```python
from build123d import *

# Parameters (mm, degrees)
BOSS_EXTRUDE1_DEPTH = 1.5875
CUT_EXTRUDE2_DEPTH  = 93.054574745
FILLET1_R           = 2.54
FILLET2_R           = 1.27
FILLET3_R           = 0.508
FILLET4_R           = 0.508
BOSS_EXTRUDE3_DEPTH = 1.5875
FILLET5_R           = 1.27
FILLET6_R           = 0.254
BOSS_EXTRUDE4_DEPTH = 1.5875
CUT_EXTRUDE1_REACH  = 94.055
FILLET9_R           = 1.27
FILLET10_R          = 0.381
FILLET12_R          = 1.27
FILLET13_R          = 0.508


with BuildPart() as part:
    # Sketch1 → Boss-Extrude1 (new body)
    with BuildSketch(Plane(origin=(0, 0, 0), x_dir=(0, 0, -1), z_dir=(1, 0, 0))):
        with BuildLine():
            Line((62.185099246, -6.2738), (85.344, -14.722370106))
            Line((85.344, -14.722370106), (88.3158, -14.722370106))
            ThreePointArc((88.3158, -14.722370106), (90.111851224, -13.978421331), (90.8558, -12.182370106))
            Line((90.8558, -12.182370106), (90.8558, -12.131570106))
            Line((90.8558, -12.131570106), (89.3826, -10.658370106))
            Line((89.3826, -10.658370106), (88.9508, -10.658370106))
            Line((88.9508, -10.658370106), (88.9508, -12.182370106))
            Line((88.9508, -12.182370106), (87.376, -12.182370106))
            Line((87.376, -12.182370106), (87.376, -10.277370106))
            Line((87.376, -10.277370106), (85.344, -10.277370106))
            Line((85.344, -10.277370106), (85.344, -11.477881212))
            Line((85.344, -11.477881212), (71.07876946, -6.2738))
            Line((71.07876946, -6.2738), (87.376, -6.2738))
            Line((87.376, -6.2738), (87.376, 6.867629894))
            Line((87.376, 6.867629894), (88.9508, 6.867629894))
            Line((88.9508, 6.867629894), (88.9508, 5.089629894))
            Line((88.9508, 5.089629894), (89.9668, 5.089629894))
            ThreePointArc((89.9668, 5.089629894), (90.595417928, 5.350011965), (90.8558, 5.978629894))
            Line((90.8558, 5.978629894), (90.8558, 6.359629894))
            ThreePointArc((90.8558, 6.359629894), (90.111851224, 8.155681118), (88.3158, 8.899629894))
            Line((88.3158, 8.899629894), (85.344, 8.899629894))
            Line((85.344, 8.899629894), (62.185099246, 2.453000952))
            Line((62.185099246, 2.453000952), (-5.3213, 6.613676867))
            Line((-5.3213, 6.613676867), (-5.3213, 8.924406911))
            Line((-5.3213, 8.924406911), (-7.8613, 8.924406911))
            Line((-7.8613, 8.924406911), (-7.8613, 4.225406911))
            Line((-7.8613, 4.225406911), (-3.7338, 3.971013401))
            Line((-3.7338, 3.971013401), (-3.7338, 3.488413401))
            Line((-3.7338, 3.488413401), (-1.331252938, 3.488413401))
            ThreePointArc((-1.331252938, 3.488413401), (3.7338, 0), (-1.331252938, -3.488413401))
            Line((-1.331252938, -3.488413401), (-3.7338, -3.488413401))
            Line((-3.7338, -3.488413401), (-3.7338, -3.7338))
            Line((-3.7338, -3.7338), (-5.3213, -3.7338))
            Line((-5.3213, -3.7338), (-7.8613, -3.7338))
            Line((-7.8613, -3.7338), (-7.8613, -8.4328))
            Line((-7.8613, -8.4328), (-5.3213, -8.4328))
            Line((-5.3213, -8.4328), (-5.3213, -6.2738))
            Line((-5.3213, -6.2738), (62.185099246, -6.2738))
        make_face()
        Polygon((12.4587, -3.7338), (6.2738, -3.7338), (6.2738, 3.354206983), (12.4587, 2.973008093), align=None, mode=Mode.SUBTRACT)
        Polygon((14.3637, -4.3688), (14.3637, 3.495415512), (37.420099246, 2.074362011), (37.420099246, -4.3688), align=None, mode=Mode.SUBTRACT)
        Polygon((64.471099246, -4.3688), (64.471099246, 0.407106085), (85.344, -0.879370106), (85.344, -4.3688), align=None, mode=Mode.SUBTRACT)
        Polygon((39.325099246, -4.3688), (39.325099246, 1.956949622), (62.185099246, 0.548000952), (62.185099246, -4.3688), align=None, mode=Mode.SUBTRACT)
        Polygon((85.344, 6.922200335), (85.344, 1.025629894), (68.00108793, 2.094539469), align=None, mode=Mode.SUBTRACT)
    extrude(amount=BOSS_EXTRUDE1_DEPTH)

    # Sketch7 → Cut-Extrude2 (cut, through all)
    with BuildSketch(Plane.ZY):
        Polygon((6.5913, 8.924406911), (7.8613, 5.495406911), (7.8613, 8.924406911), align=None)
        Polygon((6.5913, -8.4328), (7.8613, -5.0038), (7.8613, -8.4328), align=None)
    extrude(amount=-CUT_EXTRUDE2_DEPTH, mode=Mode.SUBTRACT)

    # Fillet1
    fillet1_edges = [part.edges().sort_by_distance(p)[0] for p in [
        (0.79375, 2.453000952, -62.185099246),
        (0.79375, 8.899629894, -85.344),
        (0.79375, -14.722370106, -85.344),
        (0.79375, -6.2738, -62.185099246),
    ]]
    fillet(fillet1_edges, radius=FILLET1_R)

    # Fillet2
    fillet2_edges = [part.edges().sort_by_distance(p)[0] for p in [
        (0.79375, -4.3688, -85.344),
        (0.79375, -0.879370106, -85.344),
        (0.79375, 0.407106085, -64.471099246),
        (0.79375, -4.3688, -64.471099246),
        (0.79375, 1.025629894, -85.344),
        (0.79375, 6.922200335, -85.344),
        (0.79375, -4.3688, -37.420099246),
        (0.79375, 2.074362011, -37.420099246),
        (0.79375, 3.495415512, -14.3637),
        (0.79375, -4.3688, -14.3637),
        (0.79375, -4.3688, -62.185099246),
        (0.79375, 0.548000952, -62.185099246),
        (0.79375, -3.7338, -12.4587),
        (0.79375, 2.973008093, -12.4587),
        (0.79375, 3.354206983, -6.2738),
        (0.79375, -3.7338, -6.2738),
    ]]
    fillet(fillet2_edges, radius=FILLET2_R)

    # Fillet3
    fillet3_edges = [part.edges().sort_by_distance(p)[0] for p in [
        (0.79375, -6.2738, -71.07876946),
        (0.79375, -11.477881212, -85.344),
    ]]
    fillet(fillet3_edges, radius=FILLET3_R)

    # Fillet4
    fillet4_edges = [part.edges().sort_by_distance(p)[0] for p in [
        (0.79375, -10.277370106, -85.344),
    ]]
    fillet(fillet4_edges, radius=FILLET4_R)

    # Sketch6 → Boss-Extrude3 (add)
    with BuildSketch(Plane.ZY.offset(-1.5875)):
        Polygon((-47.9467, -6.2738), (-47.0577, -6.2738), (-47.9467, -7.1628), align=None)
        Polygon((-49.5342, -6.2738), (-50.4232, -6.2738), (-49.5342, -7.1628), align=None)
        Polygon((-49.5342, 3.232723947), (-50.421516262, 3.178035274), (-49.5342, 4.121723947), align=None)
        Polygon((-47.059383738, 3.385256278), (-47.9467, 4.219567605), (-47.9467, 3.330567605), align=None)
        Polygon((-47.9467, 4.219567605), (-47.9467, 3.330567605), (-47.059383738, 3.385256278), align=None)
        Polygon((-49.5342, 4.121723947), (-49.5342, 3.232723947), (-50.421516262, 3.178035274), align=None)
        Polygon((-50.4232, -6.2738), (-49.5342, -7.1628), (-49.5342, -6.2738), align=None)
        Polygon((-47.9467, -7.1628), (-47.9467, -6.2738), (-47.0577, -6.2738), align=None)
    extrude(amount=BOSS_EXTRUDE3_DEPTH)

    # Fillet5
    fillet5_edges = [part.edges().sort_by_distance(p)[0] for p in [
        (0.79375, 3.385256278, -47.059383738),
        (0.79375, 3.178035274, -50.421516262),
        (0.79375, -6.2738, -50.4232),
        (0.79375, -6.2738, -47.0577),
    ]]
    fillet(fillet5_edges, radius=FILLET5_R)

    # Fillet6
    fillet6_edges = [part.edges().sort_by_distance(p)[0] for p in [
        (0.79375, 4.219567605, -47.9467),
        (0.79375, 4.121723947, -49.5342),
        (0.79375, -7.1628, -49.5342),
        (0.79375, -7.1628, -47.9467),
    ]]
    fillet(fillet6_edges, radius=FILLET6_R)

    # Sketch4 → Boss-Extrude4 (add)
    with BuildSketch(Plane(origin=(1.5875, 0, 0), x_dir=(0, 0, -1), z_dir=(1, 0, 0))):
        with BuildLine():
            Line((39.325099246, 1.956949622), (43.194043845, 1.718491864))
            ThreePointArc((43.194043845, 1.718491864), (39.961542096, -1.228517825), (43.006630195, -4.3688))
            Line((43.006630195, -4.3688), (39.325099246, -4.3688))
            Line((39.325099246, -4.3688), (39.325099246, 1.956949622))
        make_face()
    extrude(amount=-BOSS_EXTRUDE4_DEPTH)

    # Sketch5 → Cut-Extrude1 (cut, up to next)
    with BuildSketch(Plane(origin=(1.5875, 0, 0), x_dir=(0, 0, -1), z_dir=(1, 0, 0)), mode=Mode.PRIVATE) as cut_extrude1_sk1:
        Polygon((3.7592, -4.445), (3.7592, -4.953), (5.3467, -4.953), (5.3467, -4.445), (5.3467, -3.683), (5.3467, -3.175), (3.7592, -3.175), (3.7592, -3.683), align=None)
    cut_extrude1_tool1 = extrude(cut_extrude1_sk1.sketch, amount=-CUT_EXTRUDE1_REACH, mode=Mode.PRIVATE) & part.part
    add(cut_extrude1_tool1.solids().sort_by_distance((1.5875, -4.064, -4.55295))[0], mode=Mode.SUBTRACT)

    # Fillet9
    fillet9_edges = [part.edges().sort_by_distance(p)[0] for p in [
        (0.79375, 3.488413401, 1.331252938),
        (0.79375, -3.488413401, 1.331252938),
    ]]
    fillet(fillet9_edges, radius=FILLET9_R)

    # Fillet10
    fillet10_edges = [part.edges().sort_by_distance(p)[0] for p in [
        (0.79375, 2.094539469, -68.00108793),
    ]]
    fillet(fillet10_edges, radius=FILLET10_R)

    # Fillet12
    # the kernel refuses this fillet: 1.27 mm, written as the material it takes off along each edge
    with BuildSketch(Plane(origin=(-0.569074331, -5.0038, 7.8613), x_dir=(0, 1, 0), z_dir=(1, 0, 0))) as fillet12_piece_1:
        with BuildLine():
            CenterArc((FILLET12_R * 0.179236009778, -FILLET12_R), FILLET12_R, 90, 20.32313683)
            Line((-FILLET12_R * 0.168078346046, -FILLET12_R * 0.0622512392763), (0, 0))
            Line((0, 0), (FILLET12_R * 0.179236009778, 0))
        make_face()
    extrude(amount=2.725648662, mode=Mode.SUBTRACT)
    with BuildSketch(Plane(origin=(-3.175, -3.7338, 7.8613), x_dir=(0, 1.571796061637141e-12, -1.0), z_dir=(1, 0, 0))) as fillet12_piece_2:
        with BuildLine():
            CenterArc((FILLET12_R, -FILLET12_R), FILLET12_R, 90, 90)
            Line((0, -FILLET12_R), (0, 0))
            Line((0, 0), (FILLET12_R, 0))
        make_face()
    extrude(amount=7.9375, mode=Mode.SUBTRACT)
    with BuildSketch(Plane(origin=(-0.569074331, 5.495406911, 7.8613), x_dir=(0, -1, 0), z_dir=(1, 0, 0))) as fillet12_piece_3:
        with BuildLine():
            CenterArc((FILLET12_R * 0.179236009778, FILLET12_R), FILLET12_R, 249.67686317, 20.32313683)
            Line((-FILLET12_R * 0.168078346046, FILLET12_R * 0.0622512392763), (0, 0))
            Line((0, 0), (FILLET12_R * 0.179236009778, 0))
        make_face()
    extrude(amount=2.725648662, mode=Mode.SUBTRACT)
    with BuildSketch(Plane(origin=(-2.985337445, 4.225406911, 7.8613), x_dir=(0, -0.06151706759749907, -0.9981060316390262), z_dir=(1, 0, 0))) as fillet12_piece_4:
        with BuildLine():
            CenterArc((FILLET12_R * 0.940263762219, FILLET12_R), FILLET12_R, 183.526895232, 86.473104768)
            Line((-FILLET12_R * 0.0578422694199, FILLET12_R * 0.938482932403), (0, 0))
            Line((0, 0), (FILLET12_R * 0.940263762219, 0))
        make_face()
    extrude(amount=7.55817489, mode=Mode.SUBTRACT)

    # Fillet13
    fillet13_edges = [part.edges().sort_by_distance(p)[0] for p in [
        (0.79375, 8.924406911, 6.5913),
        (0.79375, -8.4328, 6.5913),
    ]]
    fillet(fillet13_edges, radius=FILLET13_R)


solid = part.part
```
The listing builds one solid part. Answer for the finished solid, in the listing's coordinates (mm). A direction names the side the tool comes from. Give positions to 0.01 mm unless a question says otherwise; leave off trailing zeros. Loops run counter-clockwise (first coordinate to the right, second up) from the corner with the lowest first, then second, coordinate; pieces in that order, holes last. Notation, with made-up numbers: M 68,46.25 L 107,46.25 A17 ccw 107,73.25 Z; hole C 55.25,-29.5 d4. An arc over 180 degrees is marked long. One line per item, written item: value.
Q1. For faces 3 (the face through (1, -10.277, -87)), 4 (the face through (0.78, 4.56, -76.86)), 5 (the face through (1, -6.274, -56)), 6 (the face through (1, -3.488, 3)), determine the directions among +Z, -Z, +X, -X, +Y, -Y from which every point of the face is accessible in a straight line to the end or side of a thin tool.
Working result:
face 3: -Z, +X, -X
face 4: +X, -X
face 5: +X, -X, -Y
face 6: +Z, +X, -X
Q2. A cutting plane is placed at D-D on y = -9.25. Determine the outline of the cut face in (x, z).
Working result:
outline: M 0,-79.24 L 1.59,-79.24 L 1.59,-70.34 L 0,-70.34 Z
Q3. A cutting plane is placed at C-C on x = 0.8. Give the number of separate pieces and of enclosed holes in the cut face, then the cut area to 3 significant figures.
Working result:
separate pieces: 1
enclosed holes: 6
area: 624 mm^2
Q4. Determine the mould class of faces 1 (the face through (1, -1, -37.42)), 2 (the face through (0.78, -14, -90.09)) for opening direction Y: +Y half, -Y half, draft (parallel to the pull), parting line (faces both ways), or undercut.
Working result:
face 1: undercut
face 2: -Y half
Q5. A cutting plane is placed at A-A on z = -82. Determine the outline of the cut face in (x, y), then the cut area to 3 significant figures.
Working result:
outline: M 0,-13.5 L 1.59,-13.5 L 1.59,-10.26 L 0,-10.26 Z; M 0,-6.27 L 1.59,-6.27 L 1.59,-4.37 L 0,-4.37 Z; M 0,-0.67 L 1.59,-0.67 L 1.59,1.23 L 0,1.23 Z; M 0,5.99 L 1.59,5.99 L 1.59,7.97 L 0,7.97 Z
area: 14.3 mm^2
Q6. Find the intervals of material crossed by line 1 (Y direction, x = 0.55, z = -77); line 2 (Z direction, x = 1, y = -2.25); line 3 (Y direction, x = 0.75, z = -53), in increasing order. Write a range as from..to.
Working result:
line 1: y = -11.68..-8.43, -6.27..-4.37, -0.37..1.54, 4.6..6.58
line 2: z = -87.38..-85.34, -64.47..-62.19, -40.1..-37.42, -14.36..-12.46, -6.27..-2.98
line 3: y = -6.27..-4.37, 1.11..3.02
Q7. Flat-ended cylindrical pins translate along their axes: P1, Ø0.7, axis at x = 0.5, z = 5.5, coming from the -Y side; P2, Ø0.8, axis at x = 0.5, z = -9.5, coming from the +Y side; P3, Ø0.8, axis at x = 0.5, z = -31, coming from the -Y side. Find the tip coordinate at first contact, or state that the pin passes through.
Working result:
P1: stops at y = -8.43
P2: stops at y = 5.72
P3: stops at y = -6.27
Q8. A cutting plane is placed at B-B on z = -2.5. Determine the outline of the cut face in (x, y).
Working result:
outline: M 0,-6.27 L 1.59,-6.27 L 1.59,-2.77 L 0,-2.77 Z; M 0,2.77 L 1.59,2.77 L 1.59,6.13 L 0,6.13 Z
